Can you work these out from the drawing? Everything is in mm from the part's minimum corner. A direction names the side the tool comes from. Round coordinates to 2 decimals unless told otherwise and drop trailing zeros. Loops run counter-clockwise (first coordinate to the right, second up) from the corner with the lowest first, then second, coordinate; pieces in that order, holes last. Notation, with made-up numbers: (20, -11) - (75, -11) arc R22 ccw to (75, -4) - close; hole circle Ø10 at (36, -32.5). An arc over 180 degrees is marked (long way). Return JSON: item names as keys, results as strings. Group by question number.
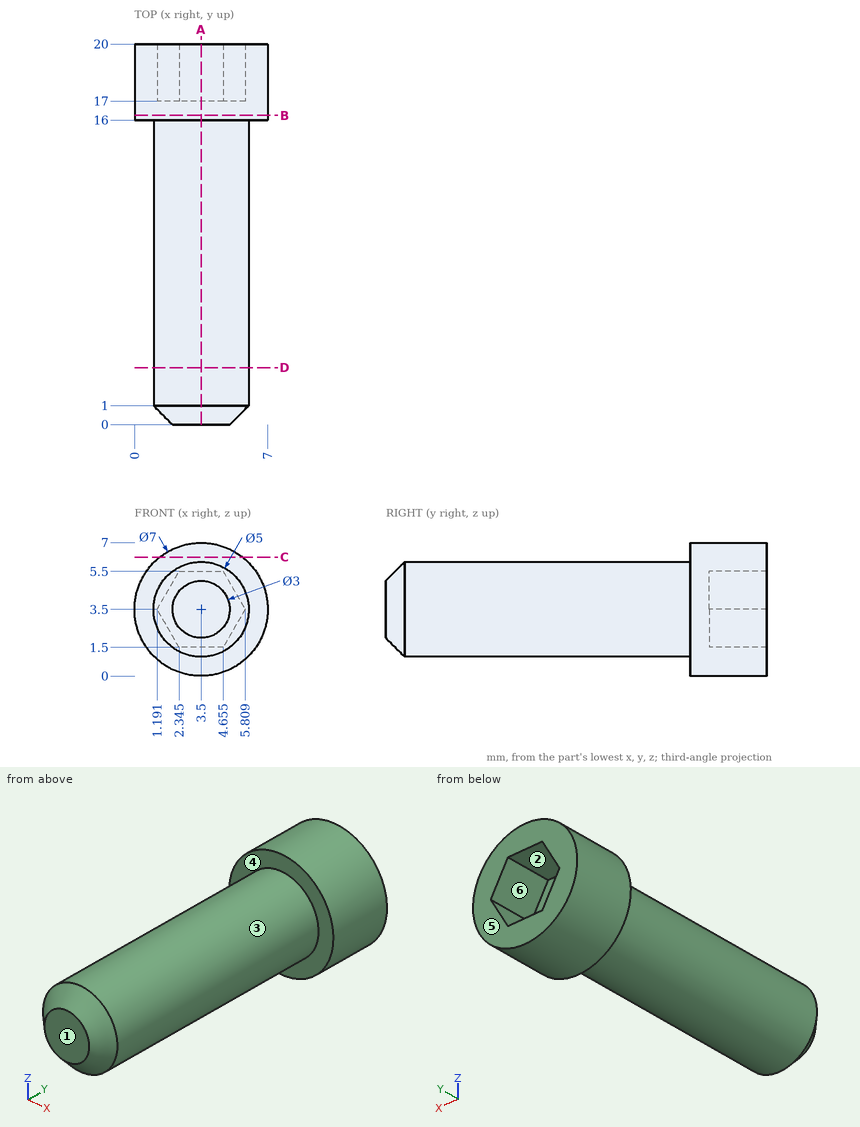
Q1. Imagine slicing it at B-B, the plane y = 16.25. List the corners of the cut face in (x, z) for me, and give its area (3 significant figures).
Q2. For the marked faces 4, 5 and 6, which set-ups out of +Z, -Z, +X, -X, +Y, -Y let a thin tool reach every point of the face, with its end or its side?
Q3. Will these pins go through, and if not, where does the flat tip stop? pin 1 Ø0.7 at (x, y) = (4, 19) entering from +Z; pin 2 Ø1.5 at (x, z) = (4.5, 6) entering from -Y; pin 3 Ø1.2 at (x, z) = (3.5, 4.5) entering from +Y.
Q4. Imagine slicing it at C-C, the plane z = 6.25. List the corners of the cut face in (x, y) for me (1 decimal).
Q5. Please list where these lines run through material, in increasing order: line 1 (Z direction, x = 2, y = 15.25); line 2 (Z direction, x = 1.75, y = 18.5); line 3 (Y direction, x = 3, z = 3).
Q6. If we mould it in two halves opening along X, with no side actions, what happens to the marked faces 1, 2 and 3? For each: +X half, -X half, draft (parallel to the pull), parting line (faces both ways), or undercut.
Q7. Imagine slicing it at A-A, the plane x = 3.5. List the corners of the cut face in (y, z) for me.
Q8. Imagine slicing it at D-D, the plane y = 3. List the corners of the cut face in (x, z) for me.
Output values:
{
 "1": {"outline": "circle Ø7 at (3.5, 3.5)", "area": "38.5 mm^2"},
 "2": {"face 4": "-Y", "face 5": "+Z, -Z, +X, -X, +Y", "face 6": "+Y"},
 "3": {"pin 1": "stops at z = 7", "pin 2": "stops at y = 0.44", "pin 3": "stops at y = 17"},
 "4": {"outline": "(1.3, 16) - (5.7, 16) - (5.7, 20) - (1.3, 20) - close"},
 "5": {"line 1": "z = 1.5 to 5.5", "line 2": "z = 0.47 to 2.53, 4.47 to 6.53", "line 3": "y = 0 to 17"},
 "6": {"face 1": "draft", "face 2": "undercut", "face 3": "parting line"},
 "7": {"outline": "(0, 2) - (1, 1) - (16, 1) - (16, 0) - (20, 0) - (20, 1.5) - (17, 1.5) - (17, 5.5) - (20, 5.5) - (20, 7) - (16, 7) - (16, 6) - (1, 6) - (0, 5) - close"},
 "8": {"outline": "circle Ø5 at (3.5, 3.5)"}
}
